Verification items for this drawing (mm, ordinates from the low corner). A direction names the side the tool comes from. Round coordinates to 2 decimals unless told otherwise and drop trailing zeros. Loops run counter-clockwise (first coordinate to the right, second up) from the corner with the lowest first, then second, coordinate; pieces in that order, holes last. Notation, with made-up numbers: M 69,60 L 75,60 A17 ccw 75,86 Z; hole C 2.25,76.5 d4. An arc over 180 degrees is marked long. One line per item, written item: value.
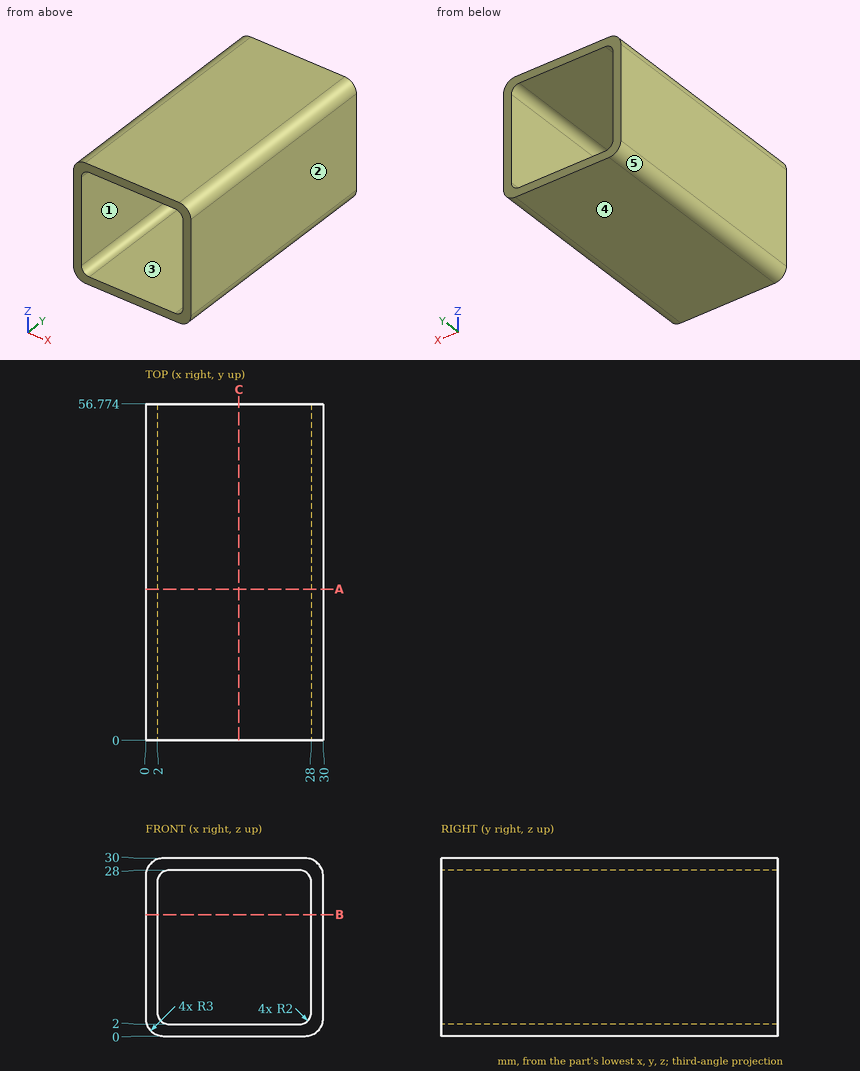
(1) Thickness scan on L1, parallel to X at y = 29, z = 15.5; L2, parallel to X at y = 19, z = 27.5. Record the ranges inside material, lowest first. Write a range as from..to.
Completed:
L1: x = 0..2, 28..30
L2: x = 0.04..2.68, 27.32..29.96
(2) Sectioned sample at C-C on x = 15.75. Enter the section's corners in (y, z), and give its area (3 significant figures).
Completed:
outline: M 0,0 L 56.77,0 L 56.77,2 L 0,2 Z; M 0,28 L 56.77,28 L 56.77,30 L 0,30 Z
area: 227 mm^2
(3) Mould release check, pull along X, two halves, no side actions. Record for the marked faces 3, 4 and 5: +X half, -X half, draft (parallel to the pull), parting line (faces both ways), or undercut.
Completed:
face 3: undercut
face 4: draft
face 5: -X half
(4) Tool access check on the marked faces 1 and 2. Record the directions out of +Z, -Z, +X, -X, +Y, -Y that give a thin tool (end or side, any length) a straight path to the whole face; none if there is none.
Completed:
face 1: +Y, -Y
face 2: +Z, -Z, +X, +Y, -Y
(5) Sectioned sample at B-B on z = 20.5. Enter the section's corners in (x, y), and give its area (3 significant figures).
Completed:
outline: M 0,0 L 2,0 L 2,56.77 L 0,56.77 Z; M 28,0 L 30,0 L 30,56.77 L 28,56.77 Z
area: 227 mm^2
(6) Sectioned sample at A-A on y = 25.5. Enter the section's corners in (x, z), and give its area (3 significant figures).
Completed:
outline: M 0,3 A3 ccw 3,0 L 27,0 A3 ccw 30,3 L 30,27 A3 ccw 27,30 L 3,30 A3 ccw 0,27 Z; hole M 2,4 A2 ccw 4,2 L 26,2 A2 ccw 28,4 L 28,26 A2 ccw 26,28 L 4,28 A2 ccw 2,26 Z
area: 220 mm^2
